Source: CAD feature listing. Evaluate the final solid. Frame: model axes, mm. Face numbers are marked on the shaded views. A direction names the side the tool comes from. Coordinates: 2 decimals unless noted, no trailing zeros. Loops run counter-clockwise (first coordinate to the right, second up) from the corner with the lowest first, then second, coordinate; pieces in that order, holes last. Notation, with made-up numbers: M 33.5,-35 L 91.5,-35 A9 ccw 91.5,-20 Z; hole C -2,-39.5 d1. An arc over 180 degrees is marked long. One line per question, with ' | ' between items. Start each with the question number.
1. Ray query, probe 1 along Z at (x, y) = (3.5, -16.5); probe 2 along Y at (x, z) = (10.5, 1.15); probe 3 along X at (y, z) = (15.5, 0.6). Return the intervals inside material, ascending.
2. Section query C-C, the plane z = 1.2. Output: boundary loops of the cut face in (x, y), and give its area (3 significant figures).
3. Access query for the marked faces 1 and 2. Directions: +Z, -Z, +X, -X, +Y, -Y. A direction counts if a zero-diameter tool reaches every point of the face in a straight line with its end or side. Return the directions, or none.
4. Section query A-A, the plane y = 9.5. Output: boundary loops of the cut face in (x, z).
5. Section query B-B, the plane x = 12.5. Output: boundary loops of the cut face in (y, z), and give its area (3 significant figures).
6. Section query D-D, the plane y = -17. Output: boundary loops of the cut face in (x, z).
```python
from build123d import *

# Parameters (mm, degrees)
EXTRUDE_1_DEPTH = 1.5
SKETCH_3_R      = 16.2
EXTRUDE_2_DEPTH = 0.1


with BuildPart() as part:
    # 草图2 → 凸台-拉伸1 (new body)
    with BuildSketch(Plane.XY):
        with BuildLine():
            Line((-6, -20.3), (6, -20.3))
            Line((6, -20.3), (7.479773249, -16.152182272))
            ThreePointArc((7.479773249, -16.152182272), (0, 17.8), (-7.479773249, -16.152182272))
            Line((-7.479773249, -16.152182272), (-6, -20.3))
        make_face()
    extrude(amount=EXTRUDE_1_DEPTH)

    # 草图3 → 凸台-拉伸2 (add)
    with BuildSketch(Plane.XY.offset(1.5)):
        Circle(SKETCH_3_R)
    extrude(amount=EXTRUDE_2_DEPTH)


solid = part.part
```
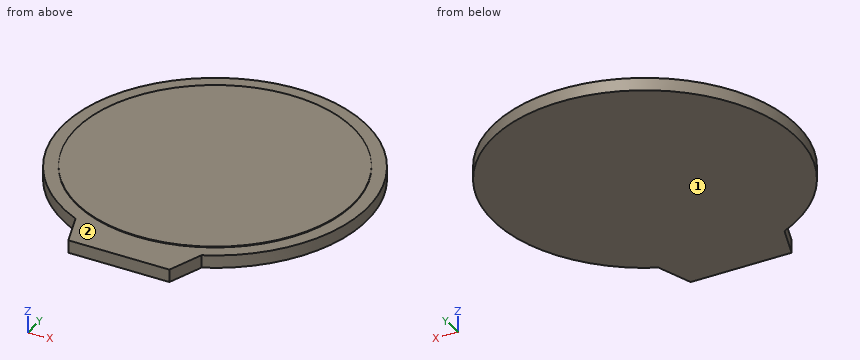
Taken from the geometry:
1) probe 1: 0 to 1.5 | probe 2: -14.37 to 14.37 | probe 3: -8.75 to 8.75
2) outline: M -7.48,-16.15 L -6,-20.3 L 6,-20.3 L 7.48,-16.15 A17.8 ccw long Z | area: 1,030 mm^2
3) face 1: -Z, +X, -X, +Y, -Y | face 2: +Z
4) outline: M -15.05,0 L 15.05,0 L 15.05,1.5 L 13.12,1.5 L 13.12,1.6 L -13.12,1.6 L -13.12,1.5 L -15.05,1.5 Z
5) outline: M -12.67,0 L 12.67,0 L 12.67,1.5 L 10.3,1.5 L 10.3,1.6 L -10.3,1.6 L -10.3,1.5 L -12.67,1.5 Z | area: 40.1 mm^2
6) outline: M -7.18,0 L 7.18,0 L 7.18,1.5 L -7.18,1.5 Z
